Source: three-view drawing plus pictorial views. Frame: mm from the lowest corner of the part. A direction names the side the tool comes from. Round coordinates to 2 decimals unless told otherwise and drop trailing zeros. Loops run counter-clockwise (first coordinate to the right, second up) from the corner with the lowest first, then second, coordinate; pieces in that order, holes last. Notation, with made-up numbers: M 0,-33 L 26,-33 A26 cw 26,-1 Z; hole C 65,43.25 d5. An arc over 180 degrees is marked long. Return JSON: item names as keys, results as strings. Group by question number.
1) Access query for the marked faces 1, 2 and 3. Directions: +Z, -Z, +X, -X, +Y, -Y. A direction counts if a zero-diameter tool reaches every point of the face in a straight line with its end or side. Return the directions, or none.
2) Material intervals for line 1 (Y direction, x = 15, z = 10); line 2 (Y direction, x = 28.5, z = 5); line 3 (Z direction, x = 15, y = 11.5), sorted ascending. Write a range as from..to.
3) Section D-D (x = 15). Count the separate pieces of the cut face and the enclosed holes in it, plus the area to 3 significant figures.
4) Section A-A (z = 11.5). Output: boundary loops of the cut face in (x, y).
5) Section B-B (z = 6.5). Output: boundary loops of the cut face in (x, y), plus the area to 3 significant figures.
6) Contact query for flat-ended pins moving along their axis: P1, Ø1.5, axis at y = 15, z = 14.5, coming from the -X side; P2, Ø2.5, axis at x = 12, z = 21, coming from the -Y side (1 decimal); P3, Ø2, axis at x = 19, y = 19.5, coming from the -Z side; P4, Ø1.5, axis at x = 10.5, z = 21, coming from the +Y side. Output: stop coordinate, or through.
7) Mould query, pull axis Y, two halves, no side actions, for the marked faces 4, 5 and 6. Classes: +Y half, -Y half, draft (parallel to the pull), parting line (faces both ways), or undercut.
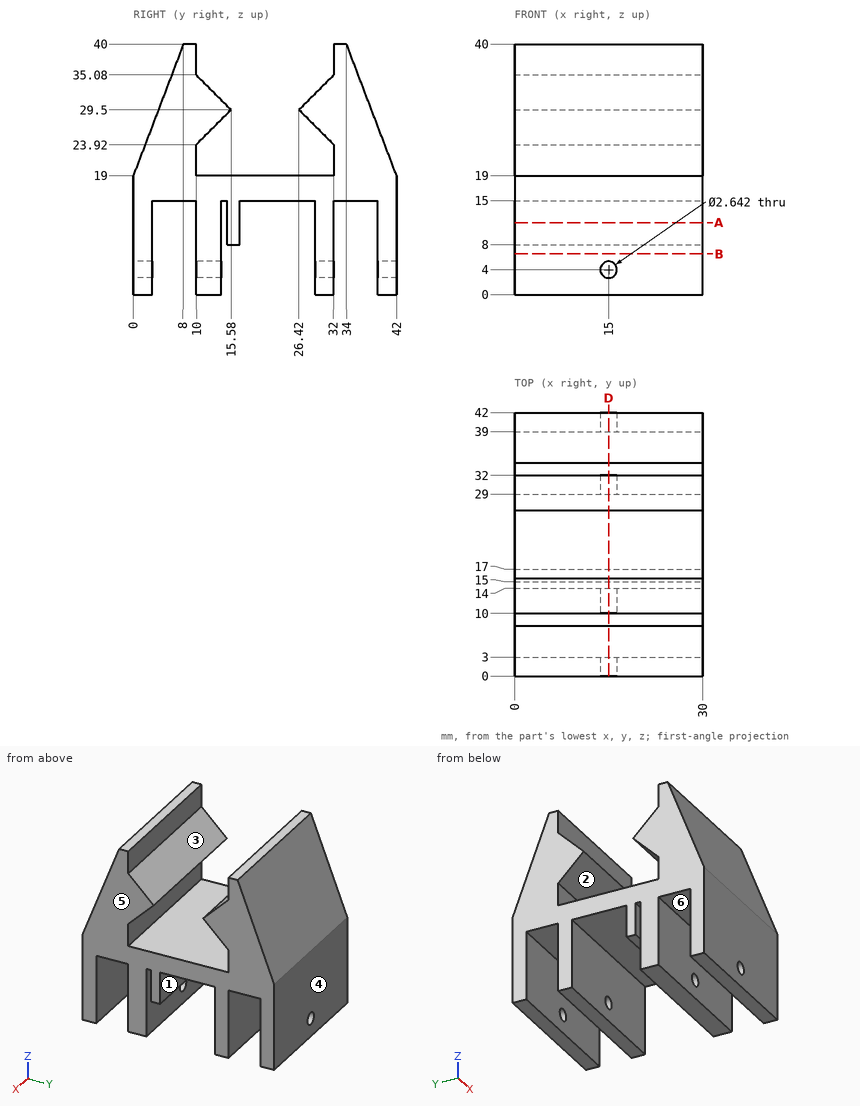
Returned:
{
 "1": {"face 1": "-Z, +X, -X", "face 2": "+X, -X", "face 3": "+Z, +X, -X"},
 "2": {"line 1": "y = 0..3, 10..14, 15..17, 29..32, 39..42", "line 2": "y = 0..3, 10..14, 29..32, 39..42", "line 3": "z = 0..2.68, 5.32..19, 25.42..33.58"},
 "3": {"separate pieces": "5", "enclosed holes": "0", "area": "657 mm^2"},
 "4": {"outline": "M 0,0 L 30,0 L 30,3 L 0,3 Z; M 0,10 L 30,10 L 30,14 L 0,14 Z; M 0,15 L 30,15 L 30,17 L 0,17 Z; M 0,29 L 30,29 L 30,32 L 0,32 Z; M 0,39 L 30,39 L 30,42 L 0,42 Z"},
 "5": {"outline": "M 0,0 L 30,0 L 30,3 L 0,3 Z; M 0,10 L 30,10 L 30,14 L 0,14 Z; M 0,29 L 30,29 L 30,32 L 0,32 Z; M 0,39 L 30,39 L 30,42 L 0,42 Z", "area": "390 mm^2"},
 "6": {"P1": "stops at x = 0", "P2": "stops at y = 0.3", "P3": "stops at z = 15", "P4": "stops at y = 41.52"},
 "7": {"face 4": "+Y half", "face 5": "draft", "face 6": "undercut"}
}
